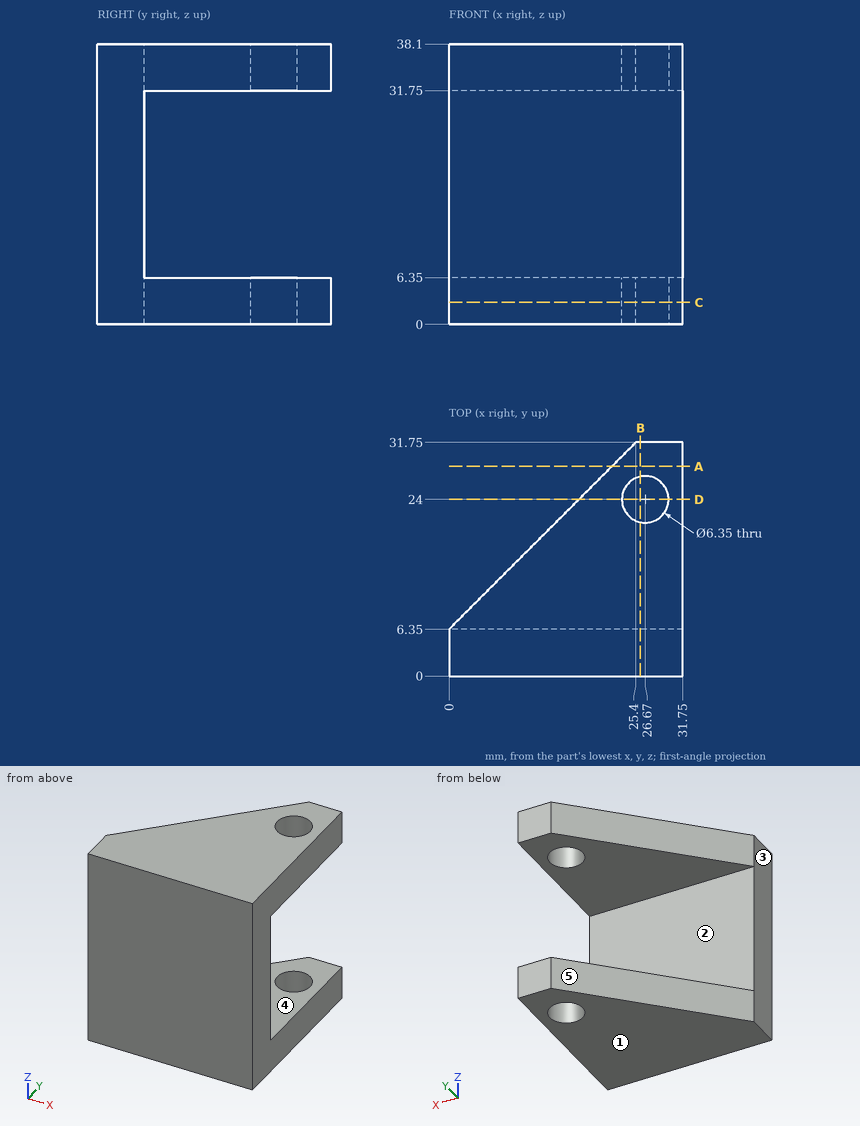
Verification items for this drawing (mm, ordinates from the low corner). A direction names the side the tool comes from. Coordinates: 2 decimals unless noted, no trailing zeros. Write each loop counter-clockwise with the first axis right and the second up, starting at its lowest first coordinate (ties: lowest second). Pieces come first, ordered by that corner, then holes. Notation, with made-up numbers: M 41,75.25 L 45,75.25 A19 cw 45,98.25 Z; hole C 34.5,-12.5 d6. An arc over 180 degrees is marked long. One line per item, written item: value. Start each with the question number.
(1) Tool access check on the marked faces 4 and 5. Record the directions out of +Z, -Z, +X, -X, +Y, -Y that give a thin tool (end or side, any length) a straight path to the whole face; none if there is none.
(2) Scan lines: line 1 along Y through (x, z) = (26.67, 35.5) (3 decimals); line 2 along Z through (x, y) = (20.5, 21.5); line 3 along Y through (x, z) = (3, 30.5). Record each from-to range of solid material in increasing order. Write a range as [from, to].
(3) Sectioned sample at C-C, the plane z = 3. Enter the section's corners in (x, y) (3 decimals).
(4) Release check for a two-part mould opening along Z. For the marked faces 1, 2 and 3 record: released by +Z, released by -Z, zero draft, split by the parting line, or undercut.
(5) Sectioned sample at D-D, the plane y = 24. Enter the section's corners in (x, z) (3 decimals).
(6) Depth check by flat-ended pin: pin 1 (3 mm diameter, centred on x = 27.5, z = 13, fed in from +Y); pin 2 (1 mm diameter, centred on x = 12.5, z = 6.5, fed in from +Y). Enter the tip coordinate at first touch or a pass-through.
(7) Sectioned sample at A-A, the plane y = 28.5. Enter the section's corners in (x, z), and give its area (3 significant figures).
(8) Sectioned sample at B-B, the plane x = 26. Enter the section's corners in (y, z).
Filled sheet:
1. face 4: +X, -X, +Y
1. face 5: +Z, -Z, -X, +Y
2. line 1: [0, 20.825], [27.175, 31.75]
2. line 2: [0, 6.35], [31.75, 38.1]
2. line 3: [0, 6.35]
3. outline: M 0,0 L 31.75,0 L 31.75,31.75 L 25.4,31.75 L 0,6.35 Z; hole C 26.67,24 d6.35
4. face 1: released by -Z
4. face 2: undercut
4. face 3: zero draft
5. outline: M 17.65,0 L 23.495,0 L 23.495,6.35 L 17.65,6.35 Z; M 17.65,31.75 L 23.495,31.75 L 23.495,38.1 L 17.65,38.1 Z; M 29.845,0 L 31.75,0 L 31.75,6.35 L 29.845,6.35 Z; M 29.845,31.75 L 31.75,31.75 L 31.75,38.1 L 29.845,38.1 Z
6. pin 1: y = 6.35
6. pin 2: y = 19.33
7. outline: M 22.15,0 L 31.75,0 L 31.75,6.35 L 22.15,6.35 Z; M 22.15,31.75 L 31.75,31.75 L 31.75,38.1 L 22.15,38.1 Z
7. area: 122 mm²
8. outline: M 0,0 L 20.9,0 L 20.9,6.35 L 6.35,6.35 L 6.35,31.75 L 20.9,31.75 L 20.9,38.1 L 0,38.1 Z; M 27.1,0 L 31.75,0 L 31.75,6.35 L 27.1,6.35 Z; M 27.1,31.75 L 31.75,31.75 L 31.75,38.1 L 27.1,38.1 Z
